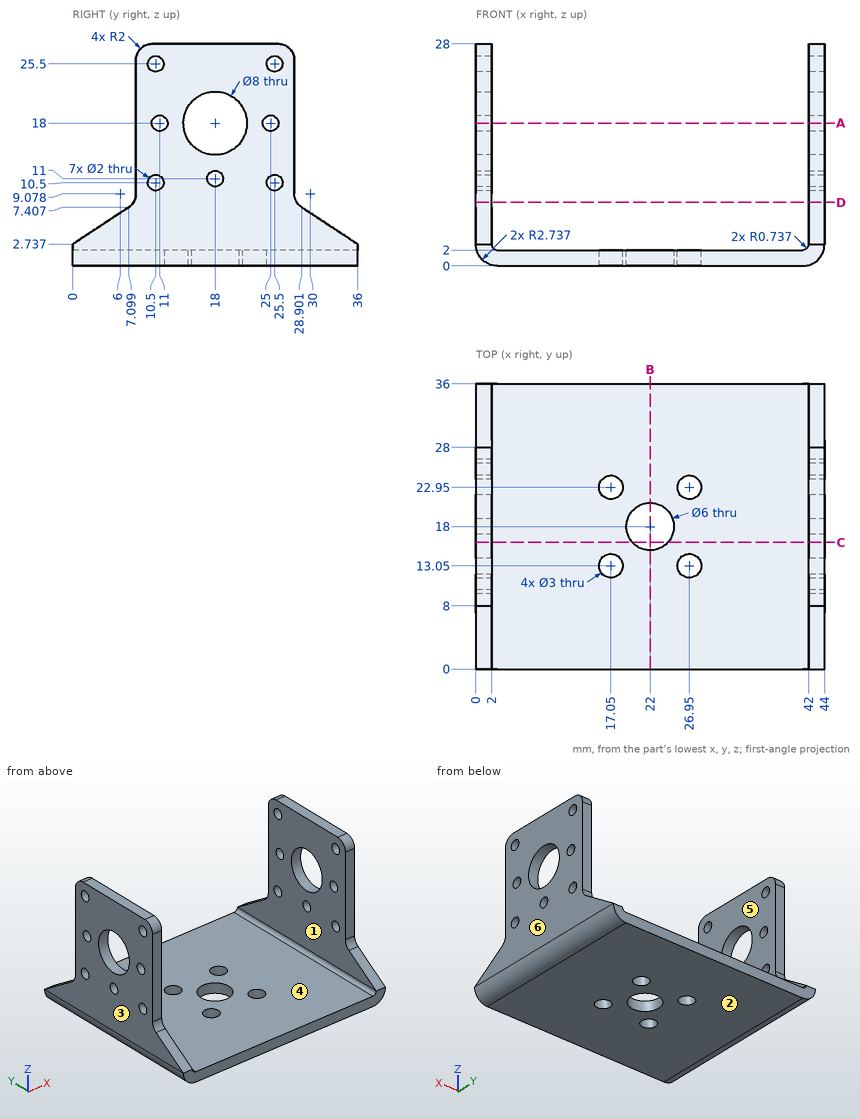
Geometry check sheet. Reference: drawing and pictorial views, mm from the part's lowest x, y, z. A direction names the side the tool comes from. Round coordinates to 2 decimals unless told otherwise and drop trailing zeros. Write each loop counter-clockwise with the first axis right and the second up, starting at its lowest first coordinate (ties: lowest second). Pieces come first, ordered by that corner, then holes. Notation, with made-up numbers: (-20.5, 57) -> (5.5, 57) arc R31 cw to (5.5, 87) -> close; hole circle Ø8 at (-27.5, 2). An arc over 180 degrees is marked (long way). Answer as CSV lines item,"result". Start each with the question number.
1) Section check C-C on y = 16. Enter the section's corners in (x, z), and give its area (3 significant figures).
2) Release check for a two-part mould opening along X. For the marked faces 3, 4, 5 and 6 record: pulls with the +X half, pulls with the -X half, needs draft (parallel to the pull), parting line crosses it, or undercut.
3) Material ranges on line 1 (Y direction, x = 1.55, z = 18); line 2 (X direction, y = 17.5, z = 22); line 3 (Y direction, x = 42.65, z = 10.5) (1 decimal), recorded low to high. Write a range as from..to.
4) Section check A-A on z = 18. State how many separate pieces and enclosed holes the cut face has.
5) Section check D-D on z = 8. Enter the section's corners in (x, y) (1 decimal).
6) Go/stop test with flat-tipped pins: P1, Ø0.6, axis at x = 43, z = 14, coming from the +Y side; P2, Ø3.5, axis at x = 26.95, y = 22.95, coming from the +Z side; P3, Ø2.5, axis at y = 18, z = 11, coming from the -X side; P4, Ø2, axis at x = 1, z = 16.5, coming from the -Y side. Record where each tip stops, or that it passes through.
7) Tool access check on the marked faces 1 and 2. Record the directions out of +Z, -Z, +X, -X, +Y, -Y that give a thin tool (end or side, any length) a straight path to the whole face; none if there is none.
8) Section check B-B on x = 22. Enter the section's corners in (y, z).
Found:
1,outline,"(0, 2.74) arc R2.74 ccw to (2.74, 0) -> (19.76, 0) -> (19.76, 2) -> (2.74, 2) arc R0.74 cw to (2, 2.74) -> (2, 14.54) -> (0, 14.54) -> close; (0, 21.46) -> (2, 21.46) -> (2, 28) -> (0, 28) -> close; (24.24, 0) -> (41.26, 0) arc R2.74 ccw to (44, 2.74) -> (44, 14.54) -> (42, 14.54) -> (42, 2.74) arc R0.74 cw to (41.26, 2) -> (24.24, 2) -> close; (42, 21.46) -> (44, 21.46) -> (44, 28) -> (42, 28) -> close"
1,area,"152 mm^2"
2,face 3,"pulls with the -X half"
2,face 4,"undercut"
2,face 5,"undercut"
2,face 6,"pulls with the +X half"
3,line 1,"y = 8..10, 12..14, 22..24, 26..28"
3,line 2,"x = 0..2, 42..44"
3,line 3,"y = 8..9.5, 11.5..17.1, 18.9..24.5, 26.5..28"
4,separate pieces,"8"
4,enclosed holes,"0"
5,outline,"(0, 7.7) -> (2, 7.7) -> (2, 28.3) -> (0, 28.3) -> close; (42, 7.7) -> (44, 7.7) -> (44, 28.3) -> (42, 28.3) -> close"
6,P1,"stops at y = 28"
6,P2,"stops at z = 2"
6,P3,"stops at x = 0"
6,P4,"stops at y = 8"
7,face 1,"+Z, +Y, -Y"
7,face 2,"-Z, +X, -X, +Y, -Y"
8,outline,"(0, 0) -> (15, 0) -> (15, 2) -> (0, 2) -> close; (21, 0) -> (36, 0) -> (36, 2) -> (21, 2) -> close"
